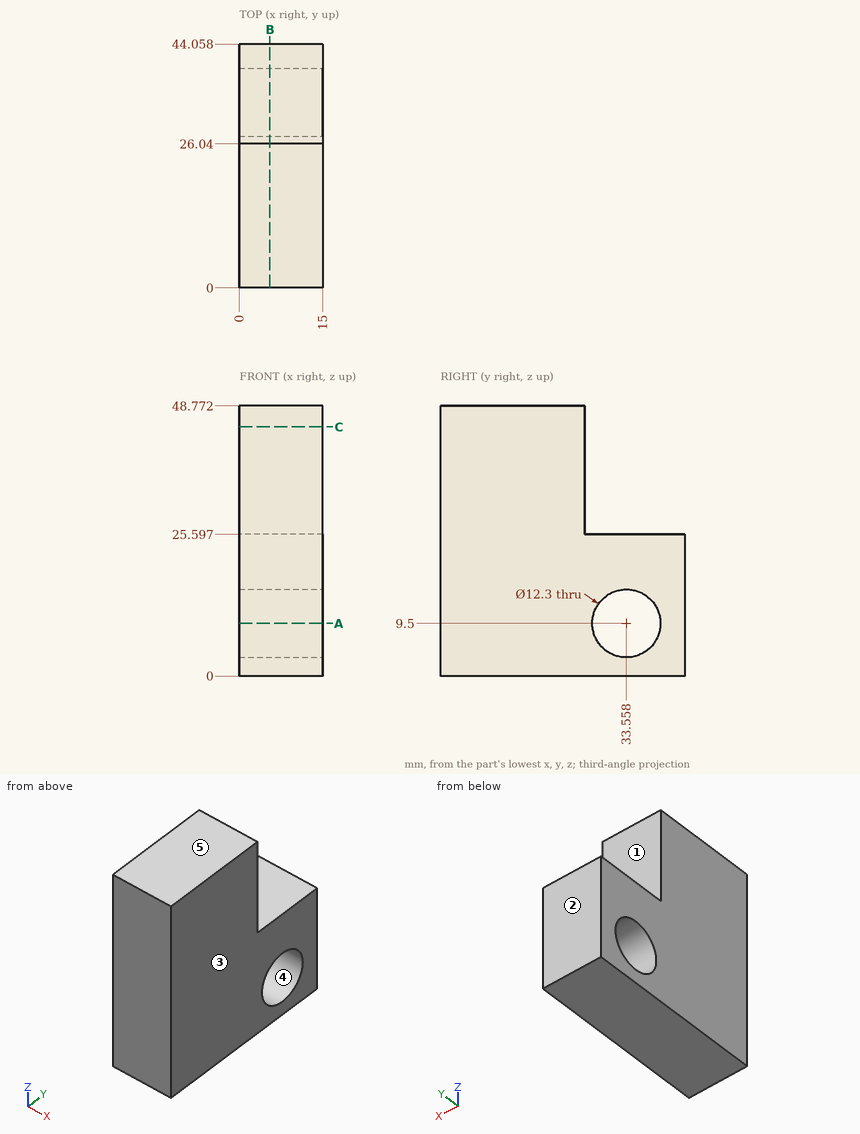
The drawing under review shows one solid part. Ordinate dimensions are in mm from its lowest x, y, z. A direction names the side the tool comes from. Round coordinates to 2 decimals unless told otherwise and drop trailing zeros. Write each loop counter-clockwise with the first axis right and the second up, starting at its lowest first coordinate (ties: lowest second). Pieces come first, ordered by that corner, then holes. Notation, with made-up numbers: (41.25, -23.75) - (98.25, -23.75) arc R18 cw to (98.25, -17.75) - close; hole circle Ø3 at (22.5, 16). An arc over 180 degrees is marked (long way). Use a Markdown table: item, result. Add a question column.
1. We need section B-B (x = 5.5). State the section outline as (y, z) points, then the cut area to 3 significant figures.
2. We need section C-C (z = 45). State the section outline as (x, y) points.
3. For the marked faces 1 and 2, list the 3-axis set-ups (+Z, -Z, +X, -X, +Y, -Y) from which the entire face can be reached by the end or side of a thin tool; tool diameter is ignored.
4. Clearance check with a flat-ended pin moving along its axis: pin 1 (4.5 mm diameter, centred on x = 4.5, z = 31.5, fed in from +Y). State where the tip first meets the part, or that it passes through.
5. We need section A-A (z = 9.5). State the section outline as (x, y) points, then the cut area to 3 significant figures.
6. Wall thickness on probe 1 along Y at (x, z) = (11.25, 9.5); probe 2 along Y at (x, z) = (7, 29); probe 3 along Z at (x, y) = (12.25, 40): over which ranges is each line inside the solid? List them lowest first.
7. Mouldability with a two-part tool opening along Z and no side actions: class the marked faces 3, 4 and 5 as +Z half, -Z half, draft (parallel to the pull), parting line (faces both ways), or undercut.
Output:
| question | item | result |
|---|---|---|
| 1 | outline | (0, 0) - (44.06, 0) - (44.06, 25.6) - (26.04, 25.6) - (26.04, 48.77) - (0, 48.77) - close; hole circle Ø12.3 at (33.56, 9.5) |
| 1 | area | 1,610 mm2 |
| 2 | outline | (0, 0) - (15, 0) - (15, 26.04) - (0, 26.04) - close |
| 3 | face 1 | +Z, +X, -X, +Y |
| 3 | face 2 | +Z, -Z, +X, -X, +Y |
| 4 | pin 1 | stops at y = 26.04 |
| 5 | outline | (0, 0) - (15, 0) - (15, 27.41) - (0, 27.41) - close; (0, 39.71) - (15, 39.71) - (15, 44.06) - (0, 44.06) - close |
| 5 | area | 476 mm2 |
| 6 | probe 1 | y = 0 to 27.41, 39.71 to 44.06 |
| 6 | probe 2 | y = 0 to 26.04 |
| 6 | probe 3 | z = 0 to 25.6 |
| 7 | face 3 | draft |
| 7 | face 4 | undercut |
| 7 | face 5 | +Z half |
